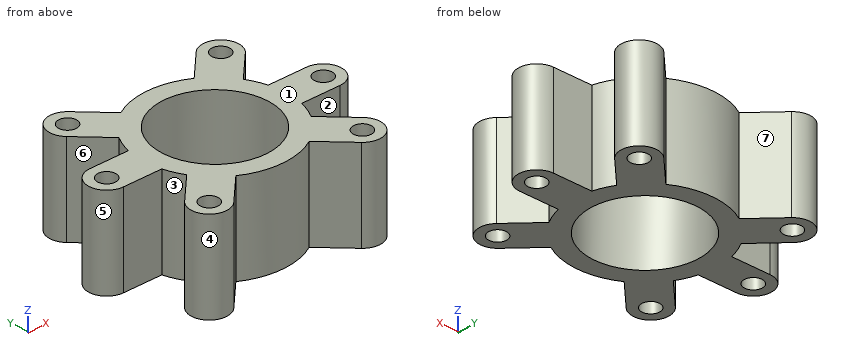
from build123d import *

# Parameters (mm, degrees)
SKETCH1_R           = 40
SKETCH1_R_2         = 30
SKETCH1_R_3         = 5
BOSS_EXTRUDE1_DEPTH = 50


with BuildPart() as part:
    # Sketch1 → Boss-Extrude1 (new body)
    # profile 1 of 7: a face of its own
    with BuildSketch(Plane.XY):
        Circle(SKETCH1_R)
        Circle(SKETCH1_R_2, mode=Mode.SUBTRACT)
    # profile 2 of 7: a face of its own
    with BuildSketch(Plane.XY):
        with BuildLine():
            ThreePointArc((-34.457195687, 20.315060063), (-28.284271247, 28.284271247), (-20.315060063, 34.457195687))
            Line((-20.315060063, 34.457195687), (-35.355339059, 49.497474683))
            ThreePointArc((-35.355339059, 49.497474683), (-49.497474683, 49.497474683), (-49.497474683, 35.355339059))
            Line((-49.497474683, 35.355339059), (-34.457195687, 20.315060063))
        make_face()
        with Locations((-42.426406871, 42.426406871)):
            Circle(SKETCH1_R_3, mode=Mode.SUBTRACT)
    # profile 3 of 7: a face of its own
    with BuildSketch(Plane.XY):
        with BuildLine():
            ThreePointArc((-38.729833462, -10), (-40, 0), (-38.729833462, 10))
            Line((-38.729833462, 10), (-60, 10))
            ThreePointArc((-60, 10), (-70, 0), (-60, -10))
            Line((-60, -10), (-38.729833462, -10))
        make_face()
        with Locations((-60, 0)):
            Circle(SKETCH1_R_3, mode=Mode.SUBTRACT)
    # profile 4 of 7: a face of its own
    with BuildSketch(Plane.XY):
        with BuildLine():
            Line((-35.355339059, -49.497474683), (-20.315060063, -34.457195687))
            ThreePointArc((-20.315060063, -34.457195687), (-28.284271247, -28.284271247), (-34.457195687, -20.315060063))
            Line((-34.457195687, -20.315060063), (-49.497474683, -35.355339059))
            ThreePointArc((-49.497474683, -35.355339059), (-49.497474683, -49.497474683), (-35.355339059, -49.497474683))
        make_face()
        with Locations((-42.426406871, -42.426406871)):
            Circle(SKETCH1_R_3, mode=Mode.SUBTRACT)
    # profile 5 of 7: a face of its own
    with BuildSketch(Plane.XY):
        with BuildLine():
            Line((49.497474683, -35.355339059), (34.457195687, -20.315060063))
            ThreePointArc((34.457195687, -20.315060063), (28.284271247, -28.284271247), (20.315060063, -34.457195687))
            Line((20.315060063, -34.457195687), (35.355339059, -49.497474683))
            ThreePointArc((35.355339059, -49.497474683), (49.497474683, -49.497474683), (49.497474683, -35.355339059))
        make_face()
        with Locations((42.426406871, -42.426406871)):
            Circle(SKETCH1_R_3, mode=Mode.SUBTRACT)
    # profile 6 of 7: a face of its own
    with BuildSketch(Plane.XY):
        with BuildLine():
            Line((60, 10), (38.729833462, 10))
            ThreePointArc((38.729833462, 10), (39.681187851, 5.040171699), (40, 0))
            ThreePointArc((40, 0), (39.681187851, -5.040171699), (38.729833462, -10))
            Line((38.729833462, -10), (60, -10))
            ThreePointArc((60, -10), (70, 0), (60, 10))
        make_face()
        with Locations((60, 0)):
            Circle(SKETCH1_R_3, mode=Mode.SUBTRACT)
    # profile 7 of 7: a face of its own
    with BuildSketch(Plane.XY):
        with BuildLine():
            ThreePointArc((20.315060063, 34.457195687), (28.284271247, 28.284271247), (34.457195687, 20.315060063))
            Line((34.457195687, 20.315060063), (49.497474683, 35.355339059))
            ThreePointArc((49.497474683, 35.355339059), (49.497474683, 49.497474683), (35.355339059, 49.497474683))
            Line((35.355339059, 49.497474683), (20.315060063, 34.457195687))
        make_face()
        with Locations((42.426406871, 42.426406871)):
            Circle(SKETCH1_R_3, mode=Mode.SUBTRACT)
    extrude(amount=BOSS_EXTRUDE1_DEPTH)


solid = part.part
For this review, take the finished solid that the model builds, in its own axes (mm). Face numbers are marked on the shaded views. A direction names the side the tool comes from. Give positions to 0.01 mm unless a question says otherwise; leave off trailing zeros. Loops run counter-clockwise (first coordinate to the right, second up) from the corner with the lowest first, then second, coordinate; pieces in that order, holes last.
Item 1: Take a section at D-D, the plane y = -24.5. State the section outline as (x, z) points, and give its area (3 significant figures).
Item 2: Take a section at A-A, the plane y = 0. State the section outline as (x, z) points, and give its area (3 significant figures).
Item 3: Tool access review of the marked faces 1, 2 and 3: name each direction out of +Z, -Z, +X, -X, +Y, -Y from which nothing blocks a thin tool from reaching the whole face with its end or side.
Item 4: Take a section at C-C, the plane z = 22.5. Give the number of separate pieces and of enclosed holes in the cut face, and give its area (3 significant figures).
Item 5: For line 1 along X through (y, z) = (0.5, 27.5); line 2 along Y through (x, z) = (-60, 11); line 3 along Y through (x, z) = (-51, 36), list the stretches that pass through material, from the lowest coordinate up.
Item 6: Take a section at B-B, the plane x = 0. State the section outline as (y, z) points.
Item 7: Insertion check: pin 1 (6 mm diameter, centred on x = 42.43, y = -42.43, fed in from -Z); pin 2 (13 mm diameter, centred on x = 60, y = 0, fed in from -Z); pin 3 (5 mm diameter, centred on x = -18, z = 19, fed in from +Y); pin 4 (2 mm diameter, centred on x = -41, z = 35.5, fed in from -Y). Each pin has a flat end and moves straight along its axis. Give the tip position at first contact, or say it passes through.
Item 8: Draft analysis for pull direction Y (two halves, no side actions). For the marked faces 4, 5, 6 and 7, state which applies: +Y half, -Y half, draft (parallel to the pull), parting line (faces both ways), or undercut.
Calculated:
1. outline: (-38.64, 0) - (-17.31, 0) - (-17.31, 50) - (-38.64, 50) - close; (17.31, 0) - (38.64, 0) - (38.64, 50) - (17.31, 50) - close
1. area: 2,130 mm2
2. outline: (-70, 0) - (-65, 0) - (-65, 50) - (-70, 50) - close; (-55, 0) - (-30, 0) - (-30, 50) - (-55, 50) - close; (30, 0) - (55, 0) - (55, 50) - (30, 50) - close; (65, 0) - (70, 0) - (70, 50) - (65, 50) - close
2. area: 3,000 mm2
3. face 1: +Z, +X, -X, +Y, -Y
3. face 2: +Z, -Z, +X
3. face 3: +Z, -Z, -X
4. separate pieces: 1
4. enclosed holes: 7
4. area: 5,120 mm2
5. line 1: x = -69.99 to -64.97, -55.03 to -30, 30 to 55.03, 64.97 to 69.99
5. line 2: y = -10 to -5, 5 to 10
5. line 3: y = -47.57 to -37.28, -10 to 10, 37.28 to 47.57
6. outline: (-40, 0) - (-30, 0) - (-30, 50) - (-40, 50) - close; (30, 0) - (40, 0) - (40, 50) - (30, 50) - close
7. pin 1: passes through
7. pin 2: stops at z = 0
7. pin 3: stops at y = 36.87
7. pin 4: stops at y = -52.42
8. face 4: undercut
8. face 5: parting line
8. face 6: undercut
8. face 7: +Y half
